Part model, mm, in its own coordinate system. Round coordinates to 2 decimals unless told otherwise and drop trailing zeros. Loops run counter-clockwise (first coordinate to the right, second up) from the corner with the lowest first, then second, coordinate; pieces in that order, holes last. Notation, with made-up numbers: M 40.25,75.5 L 67.25,75.5 A22 ccw 67.25,87.5 Z; hole C 32.25,41 d4. An arc over 180 degrees is marked long. Put each result on its own line as item: value. Start each with the question number.
1) Slice it at A-A on y = 15. Give the cut face in (x, z).
2) Probe line 1 along Y through (x, z) = (-0.5, -0.25); line 2 along Z through (x, y) = (0.25, 31); line 3 along X through (y, z) = (12.5, -2.75). List the from-to ranges inside material, lowest first.
3) Drop flat-ended pins along their axis: pin 1 Ø1 at (x, y) = (-3, 10.5) entering from -Z; pin 2 Ø1 at (x, y) = (-1.5, 26.5) entering from -Z. Give the stop position or say it passes through.
4) Pull direction X, two halves, no side cores. Call faces 1 (the flat face through (0, 0, 0)), 2 (the cylindrical face through (3.966, 21.712, -0.521)), 3 (the cylindrical face through (1.763, 35.597, 0.436)): +X half, -X half, draft (parallel to the pull), parting line (faces both ways), or undercut.
```python
from build123d import *

# Parameters (mm, degrees)
SKETCH1_R           = 4
BOSS_EXTRUDE1_DEPTH = 44
FILLET3_R           = 1.4


with BuildPart() as part:
    # Sketch1 → Boss-Extrude1 (new body)
    with BuildSketch(Plane(origin=(0, 0, 0), x_dir=(1, 0, 0), z_dir=(0, 1, 0))):
        with Locations(Location((0, 0, 0), (0, 0, 270))):
            Circle(SKETCH1_R)
    extrude(amount=BOSS_EXTRUDE1_DEPTH)

    # Fillet3
    fillet3_edges = [part.edges().sort_by_distance(p)[0] for p in [
        (0, 0, -4),
        (0, 44, -4),
    ]]
    fillet(fillet3_edges, radius=FILLET3_R)

    # Sketch6 → CSK for M3 Oval Head Machine Screw1 (revolve, cut)
    with BuildSketch(Plane(origin=(0.311679131, 35.67179677, 3.987838527), x_dir=(0.9969596318094598, 0, -0.07791978274062668), z_dir=(0, 1, 0))):
        Polygon((0, 0), (0, 8), (1.725, 8), (1.7, 7.975), (1.7, 1.45), (3.15, 0), align=None)
    revolve(axis=Axis((0.806469751, 35.67179677, 10.318532189), (-0.07791978274062668, 0, -0.9969596318094597)), mode=Mode.SUBTRACT)

    # Sketch6 at point 2 (carried to point 2, square into its face) → CSK for M3 Oval Head Machine Screw1 at 2 (revolve, cut)
    with BuildSketch(Plane(origin=(-0.477245613, 35.67179677, -3.97142753), x_dir=(-0.992856932, 0, 0.119310992), z_dir=(0, 1, 0))):
        Polygon((0, 0), (0, 8), (1.725, 8), (1.7, 7.975), (1.7, 1.45), (3.15, 0), align=None)
    revolve(axis=Axis((-1.234870411, 35.67179677, -10.276069047), (0.119310992, 0, 0.992856932)), mode=Mode.SUBTRACT)


solid = part.part
```
Recorded:
1. outline: C 0,0 d8
2. line 1: y = 0 to 34.04, 37.31 to 44
2. line 2: z = -3.99 to 3.99
2. line 3: x = -2.9 to 2.9
3. pin 1: stops at z = -3.12
3. pin 2: stops at z = -3.87
4. face 1: draft
4. face 2: parting line
4. face 3: undercut
